Job drawing, mm, ordinate dimensions from the low corner. One solid piece. A direction names the side the tool comes from. Round coordinates to 2 decimals unless told otherwise and drop trailing zeros. Loops run counter-clockwise (first coordinate to the right, second up) from the corner with the lowest first, then second, coordinate; pieces in that order, holes last.
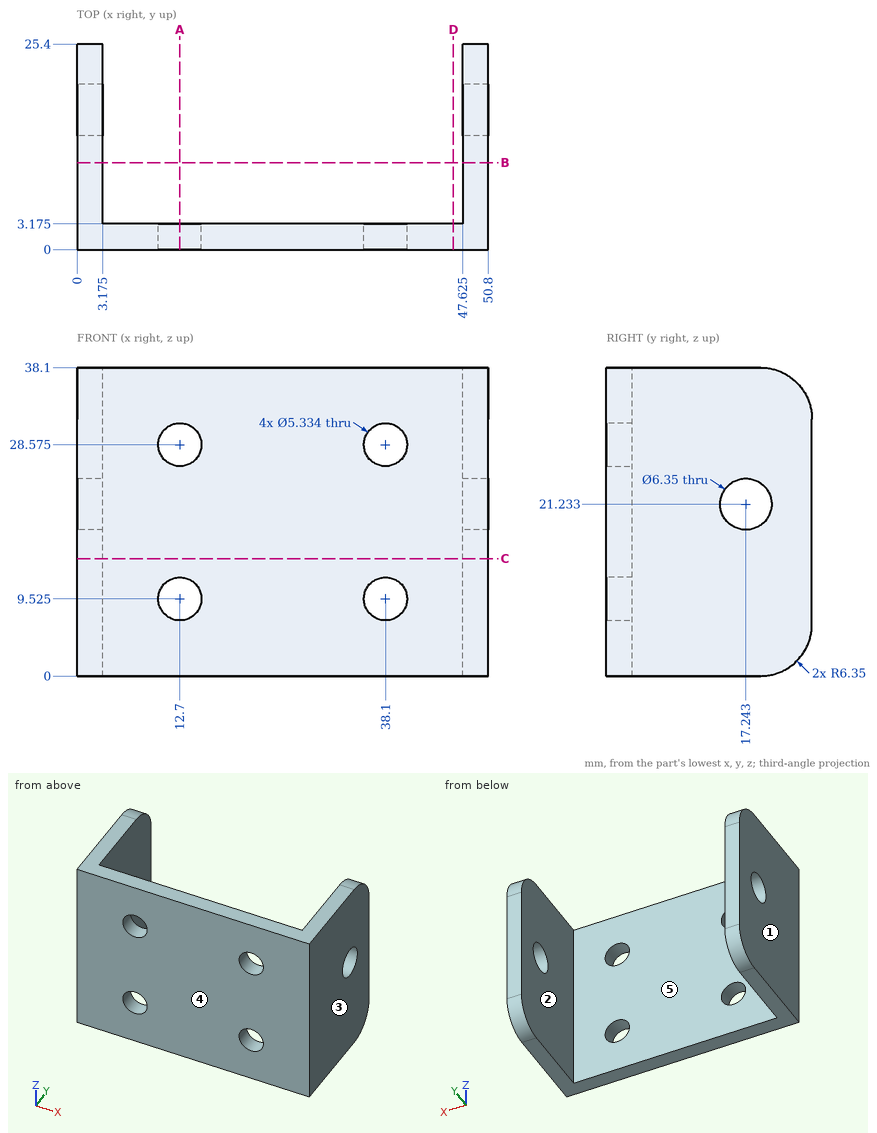
Item 1: Cut at A-A, the plane x = 12.7. Give the cut face in (y, z) (3 decimals).
Answers follow:
outline: (0, 0) - (3.175, 0) - (3.175, 6.858) - (0, 6.858) - close; (0, 12.192) - (3.175, 12.192) - (3.175, 25.908) - (0, 25.908) - close; (0, 31.242) - (3.175, 31.242) - (3.175, 38.1) - (0, 38.1) - close
Item 2: Probe line 1 (Z direction, x = 38.1, y = 1.05); line 2 (X direction, y = 17.5, z = 28) (3 decimals); line 3 (Z direction, x = 39, y = 1) (1 decimal). List the from-to ranges inside material, lowest first.
Answers follow:
line 1: z = 0 to 6.86, 12.19 to 25.91, 31.24 to 38.1
line 2: x = 0 to 3.175, 47.625 to 50.8
line 3: z = 0 to 7, 12 to 26.1, 31.1 to 38.1
Item 3: Cut at C-C, the plane z = 14.5. Give the cut face in (x, y) (3 decimals).
Answers follow:
outline: (0, 0) - (50.8, 0) - (50.8, 25.4) - (47.625, 25.4) - (47.625, 3.175) - (3.175, 3.175) - (3.175, 25.4) - (0, 25.4) - close
Item 4: 3-axis set-ups, long thin cutter, end or side, ignore diameter. For the marked faces 4 and 5: which of +Z, -Z, +X, -X, +Y, -Y reach the whole face in a straight line?
Answers follow:
face 4: +Z, -Z, +X, -X, -Y
face 5: +Z, -Z, +Y
Item 5: Flat gauge pin, fed straight in: P1, Ø3, axis at x = 43, z = 12, coming from the +Y side (3 decimals). Where does the tip first touch, or does it go through?
Answers follow:
P1: stops at y = 3.175
Item 6: Two-plate mould, pull along X, no slides. Class the marked faces 1, 2 and 3: released by +X, released by -X, zero draft, split by the parting line, or undercut.
Answers follow:
face 1: released by -X
face 2: undercut
face 3: released by +X
Item 7: Cut at B-B, the plane y = 10.75. Give the cut face in (x, z) (3 decimals), plus the area to 3 significant figures.
Answers follow:
outline: (0, 0) - (3.175, 0) - (3.175, 38.1) - (0, 38.1) - close; (47.625, 0) - (50.8, 0) - (50.8, 38.1) - (47.625, 38.1) - close
area: 242 mm2
Item 8: Cut at D-D, the plane x = 46.5. Give the cut face in (y, z) (3 decimals).
Answers follow:
outline: (0, 0) - (3.175, 0) - (3.175, 38.1) - (0, 38.1) - close
